from build123d import *

# Parameters (mm, degrees)
F1_DEPTH = 304.8
F2_T     = -10.16


# Not quite as in the source:
# - a length typed as a fraction of an inch, garbled in the dataset ("3 / 203.2 mm" for 3/8 in), is restored


with BuildPart() as f1:
    # F0 (on Top) → F1 (new body)
    with BuildSketch(Plane.XY):
        Polygon((-9.5800449151, 1.4236958328), (-38.7624735933, -14.5894044641), (-44.4378743236, -47.3891506708), (-22.332554599, -72.2766649008), (10.9077289615, -70.5111413261), (30.2523648586, -43.4220552086), (21.1344477032, -11.4080409114), align=None)
    extrude(amount=-F1_DEPTH)

    # F2
    f2_openings = [f1.faces().sort_by_distance(p)[0] for p in [
        (-7.545487, -36.881823, 0),
    ]]
    offset(amount=F2_T, openings=f2_openings)


solid = f1.part
The listing builds one solid part. Answer for the finished solid, in the listing's coordinates (mm). A direction names the side the tool comes from. Give positions to 0.01 mm unless a question says otherwise; leave off trailing zeros. Order: outer loops, then holes, each group sorted by start corner. A loop starts at its lowest first (then second) coordinate and runs counter-clockwise, first axis right, second up. Notation, with made-up numbers: (7, 74) - (39, 74) arc R15 ccw to (39, 101) - close; hole circle Ø6 at (87.5, 45). An arc over 180 degrees is marked (long way). One line per item, written item: value. Start each with the question number.
1) A cutting plane is placed at A-A on z = -95. Give the vertices of the cut face in (x, y).
2) The mould has two halves that part along Y. Classify faces 1 (the face through (-5.945, -71.406, -150.266)), 2 (the face through (-23.967, -6.471, -150.266)), 3 (the face through (2.01, -14.43, -145.26)): released by +Y, released by -Y, zero draft, split by the parting line, or undercut.
3) A tool of negligible diameter and unlimited length cuts with its end or side. For faces 4 (the face through (-6.416, -61.257, -145.258)), 5 (the face through (-33, -35, 0)), from which of +Z, -Z, +X, -X, +Y, -Y can it reach the whole face along a straight path? Write none if from no direction.
4) A cutting plane is placed at C-C on x = -26. Give the vertices of the cut face in (y, z).
5) Find the intervals of material crossed by L1, parallel to Z at x = -12, y = -58; L2, parallel to X at y = -45, z = -260.5; L3, parallel to Y at x = -5, z = -252, in increasing order.
6) A cutting plane is placed at B-B on y = -54.5. Give the vertices of the cut face in (x, z).
7) Given pin 1 Ø6 at (x, z) = (3.5, -64.5) entering from +Y; pin 2 Ø6 at (y, z) = (-30, -138) entering from -X; pin 3 Ø10 at (y, z) = (-19, -245) entering from +X, each flat-ended and moving along its own axis, determine where each tip first touches the part or whether it passes through.
Answer sheet:
1. outline: (-44.44, -47.39) - (-22.33, -72.28) - (10.91, -70.51) - (30.25, -43.42) - (21.13, -11.41) - (-9.58, 1.42) - (-38.76, -14.59) - close; hole (-33.59, -44.3) - (-17.99, -61.87) - (5.48, -60.62) - (19.14, -41.5) - (12.7, -18.9) - (-8.98, -9.84) - (-29.59, -21.14) - close
2. face 1: released by -Y
2. face 2: released by +Y
2. face 3: undercut
3. face 4: +Z
3. face 5: +Z, +X, -X, +Y, -Y
4. outline: (-68.15, -304.8) - (-7.59, -304.8) - (-7.59, 0) - (-19.18, 0) - (-19.18, -294.64) - (-52.85, -294.64) - (-52.85, 0) - (-68.15, 0) - close
5. L1: z = -304.8 to -294.64
5. L2: x = -44.02 to -32.97, 16.64 to 29.13
5. L3: y = -71.36 to -61.18, -11.5 to -0.49
6. outline: (-38.12, -304.8) - (22.34, -304.8) - (22.34, 0) - (9.86, 0) - (9.86, -294.64) - (-24.53, -294.64) - (-24.53, 0) - (-38.12, 0) - close
7. pin 1: stops at y = -2.79
7. pin 2: stops at x = -41.95
7. pin 3: stops at x = 24.72
